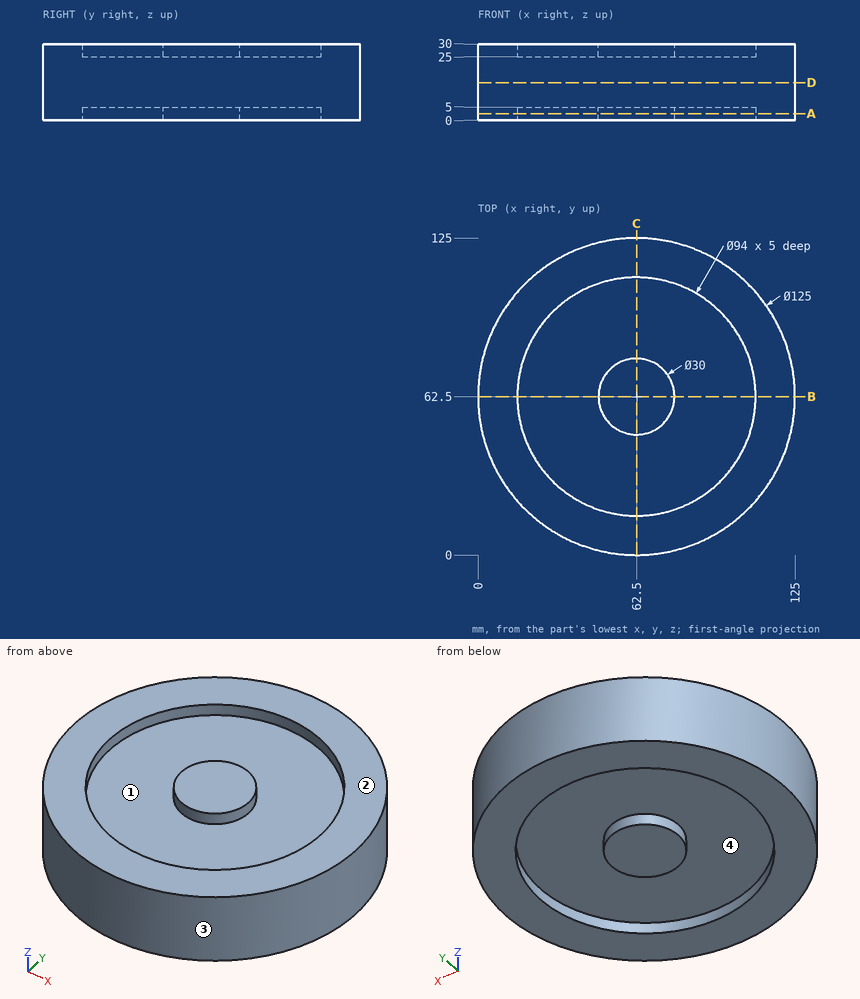
Part print with two shaded views. Sizes in mm from the minimum x, y, z corner. Give positions to 0.01 mm unless a question says otherwise; leave off trailing zeros. Order: outer loops, then holes, each group sorted by start corner. A loop starts at its lowest first (then second) coordinate and runs counter-clockwise, first axis right, second up.
(1) Mould opens along Y. For the marked faces 1, 2, 3 and 4 say: released by +Y, released by -Y, zero draft, split by the parting line, or undercut.
(2) Saw through at D-D, the plane z = 14.75. Give the cut face in (x, y).
(3) Flat gauge pins, fed straight in: pin 1 (5 mm diameter, centred on x = 69.5, y = 102, fed in from -Z); pin 2 (12 mm diameter, centred on y = 80, z = 11, fed in from -X); pin 3 (1 mm diameter, centred on x = 79, y = 84.5, fed in from +Z). Where does each tip first touch, or does it go through?
(4) Drill centre lines: L1, parallel to Y at x = 62.5, z = 27.1; L2, parallel to X at y = 61, z = 26; L3, parallel to Z at x = 66.5, y = 104.5. Where is each one in solid material? Low to high.
(5) Saw through at A-A, the plane z = 2.5. Give the cut face in (x, y), then the cut area to 3 significant figures.
(6) Saw through at B-B, the plane y = 62.5. Give the cut face in (x, z).
Results found:
1. face 1: undercut
1. face 2: zero draft
1. face 3: split by the parting line
1. face 4: undercut
2. outline: circle Ø125 at (62.5, 62.5)
3. pin 1: stops at z = 5
3. pin 2: stops at x = 1.07
3. pin 3: stops at z = 25
4. L1: y = 0 to 15.5, 47.5 to 77.5, 109.5 to 125
4. L2: x = 0.02 to 15.52, 47.58 to 77.42, 109.48 to 124.98
4. L3: z = 5 to 25
5. outline: circle Ø125 at (62.5, 62.5); circle Ø30 at (62.5, 62.5); hole circle Ø94 at (62.5, 62.5)
5. area: 6,040 mm2
6. outline: (0, 0) - (15.5, 0) - (15.5, 5) - (47.5, 5) - (47.5, 0) - (77.5, 0) - (77.5, 5) - (109.5, 5) - (109.5, 0) - (125, 0) - (125, 30) - (109.5, 30) - (109.5, 25) - (77.5, 25) - (77.5, 30) - (47.5, 30) - (47.5, 25) - (15.5, 25) - (15.5, 30) - (0, 30) - close
